Verification items for the finished model (mm, model axes). A direction names the side the tool comes from. Give positions to 0.01 mm unless a question says otherwise; leave off trailing zeros. Loops run counter-clockwise (first coordinate to the right, second up) from the corner with the lowest first, then second, coordinate; pieces in that order, holes last. Notation, with made-up numbers: M 52,70 L 101,70 A24 ccw 101,85 Z; hole C 43.5,83 d3. An arc over 180 degrees is marked long. Use a Markdown table: item, result.
from build123d import *

# Parameters (mm, degrees)
SKETCH2_R               = 2.5
SKETCH3_R               = 2.5
SKETCH4_W               = 1
SKETCH4_H               = 5
BOSS_EXTRUDE1_DEPTH     = 55
SKETCH3_7_W             = 5
SKETCH3_7_H             = 9
BOSS_EXTRUDE4_DEPTH     = 1
SKETCH8_W               = 0.6
SKETCH8_H               = 8
CUT_EXTRUDE2_DEPTH      = 1.0000001
CUT_EXTRUDE2_DEPTH_BACK = 6.0000001


with BuildPart() as part:
    # Sketch2 → Loft1 section 0
    with BuildSketch(Plane.XY):
        Circle(SKETCH2_R)
    # Sketch3 → Loft1 section 1
    with BuildSketch(Plane.XY.offset(16.5)):
        Circle(SKETCH3_R)
    loft()

    # Sketch4 → Boss-Extrude1 (add)
    with BuildSketch(Plane(origin=(0, 0, 0), x_dir=(1, 0, 0), z_dir=(0, 1, 0))):
        with Locations((0, -9.75)):
            Rectangle(SKETCH4_W, SKETCH4_H)
    extrude(amount=-BOSS_EXTRUDE1_DEPTH)

    # Sketch3_7 → Boss-Extrude4 (add)
    with BuildSketch(Plane.XY.offset(16.5)):
        Rectangle(SKETCH3_7_W, SKETCH3_7_H)
    extrude(amount=BOSS_EXTRUDE4_DEPTH)

    # Sketch8 → Cut-Extrude2 (cut, two sides)
    with BuildSketch(Plane(origin=(2.5, 0, 0), x_dir=(0, 0, -1), z_dir=(1, 0, 0))) as cut_extrude2_sk:
        with Locations((-17, 0)):
            Rectangle(SKETCH8_W, SKETCH8_H)
    extrude(amount=CUT_EXTRUDE2_DEPTH, mode=Mode.SUBTRACT)
    extrude(cut_extrude2_sk.sketch, amount=-CUT_EXTRUDE2_DEPTH_BACK, mode=Mode.SUBTRACT)


solid = part.part
(1) Cross-section at A-A on x = 0. Record the cut outline in (y, z).
Results below:
| item | result |
|---|---|
| outline | M -55,7.25 L -2.5,7.25 L -2.5,0 L 2.5,0 L 2.5,16.5 L 4.5,16.5 L 4.5,17.5 L -4.5,17.5 L -4.5,16.5 L -2.5,16.5 L -2.5,12.25 L -55,12.25 Z; hole M -4,16.7 L 4,16.7 L 4,17.3 L -4,17.3 Z |
(2) Cross-section at B-B on y = -1.5. Record the cut outline in (x, z).
Results below:
| item | result |
|---|---|
| outline | M -2.5,16.5 L -2,16.5 L -2,0 L 2,0 L 2,16.5 L 2.5,16.5 L 2.5,16.7 L -2.5,16.7 Z; M -2.5,17.3 L 2.5,17.3 L 2.5,17.5 L -2.5,17.5 Z |
(3) Draft check along Z on faces 1 (the flat face through (0, 4.5, 17)), 2 (the flat face through (0, 0, 16.7)), 3 (the flat face through (0, 0, 17.3)), 4 (the flat face through (0, 0, 0)). Enter one of: +Z half, -Z half, draft (parallel to the pull), parting line (faces both ways), or undercut.
Results below:
| item | result |
|---|---|
| face 1 | draft |
| face 2 | undercut |
| face 3 | undercut |
| face 4 | -Z half |
(4) Material ranges on line 1 (Y direction, x = -1.1, z = 16.75); line 2 (X direction, y = -35, z = 12); line 3 (Z direction, x = -1.35, y = -2.5), recorded low to high.
Results below:
| item | result |
|---|---|
| line 1 | -4.5 to -4, 4 to 4.5 |
| line 2 | -0.5 to 0.5 |
| line 3 | 16.5 to 16.7, 17.3 to 17.5 |
(5) Cross-section at C-C on y = -29. Record the cut outline in (x, z).
Results below:
| item | result |
|---|---|
| outline | M -0.5,7.25 L 0.5,7.25 L 0.5,12.25 L -0.5,12.25 Z |
(6) Cross-section at D-D on z = 10.75. Record the cut outline in (x, y), then the cut area to 3 significant figures.
Results below:
| item | result |
|---|---|
| outline | M -0.5,-55 L 0.5,-55 L 0.5,-2.45 A2.5 ccw long -0.5,-2.45 Z |
| area | 72.2 mm^2 |
(7) Gauge pin test, flat ends, axial feed: P1, Ø4, axis at y = -33, z = 10, coming from the -X side; P2, Ø3, axis at x = -0.5, y = -17.5, coming from the +Z side; P3, Ø1.5, axis at y = -37, z = 10, coming from the +X side; P4, Ø2, axis at y = -39, z = 13.5, coming from the +X side. Record the tip position at first contact, or that the pin passes through.
Results below:
| item | result |
|---|---|
| P1 | x = -0.5 |
| P2 | z = 12.25 |
| P3 | x = 0.5 |
| P4 | through |
(8) Set-up check for faces 5 (the flat face through (0, 0, 17.5)), 6 (the flat face through (0, -28, 7.25)): record each of +Z, -Z, +X, -X, +Y, -Y from which the full face is reachable in a straight line by a thin tool's end or side.
Results below:
| item | result |
|---|---|
| face 5 | +Z, +X, -X, +Y, -Y |
| face 6 | -Z, +X, -X, -Y |
